Study the drawing (mm; zero at the part's minimum x, y, z) and answer. Coordinates: 2 decimals unless noted, no trailing zeros. Order: outer loops, then holes, each group sorted by start corner. A loop starts at its lowest first (then second) coordinate and runs counter-clockwise, first axis right, second up. Notation, with made-up numbers: (66.25, 87.25) - (81.25, 87.25) arc R32 cw to (81.25, 121.25) - close; hole circle Ø4 at (-36, 21.5). An arc over 180 degrees is marked (long way). Write item = value, one per line.
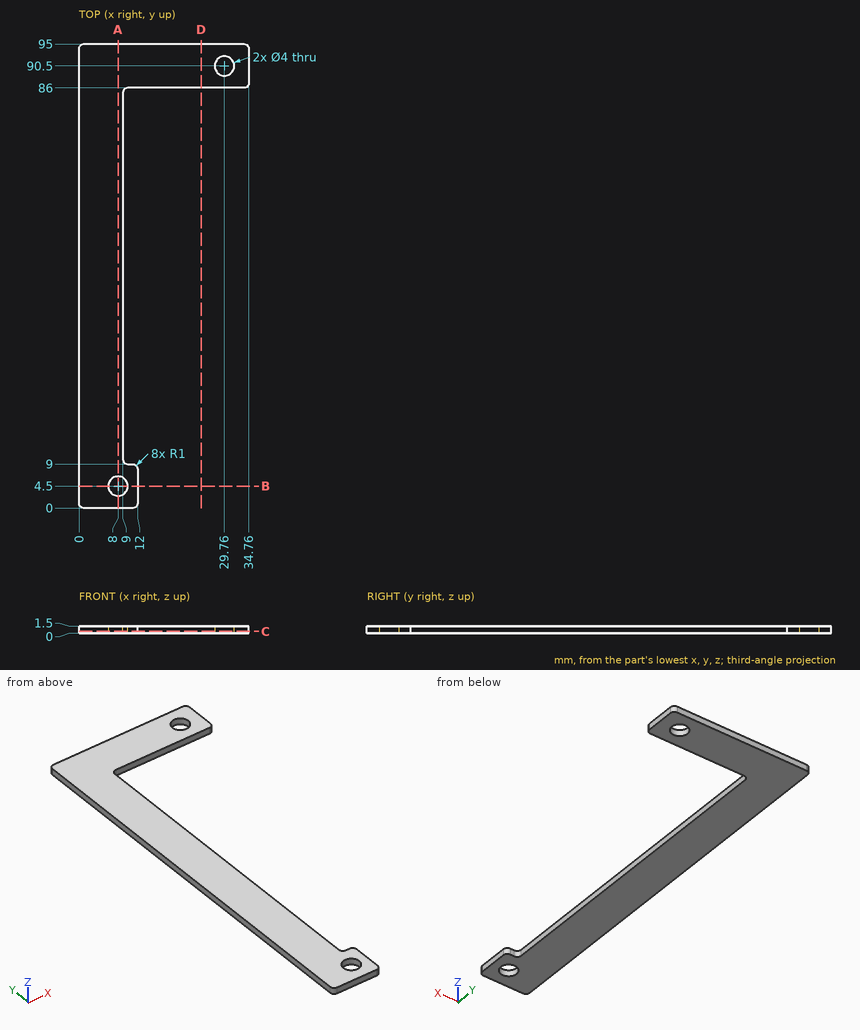
1) Straight lines are drawn through the part: line 1 along Y through (x, z) = (10.5, 0.2); line 2 along X through (y, z) = (83.5, 1.1); line 3 along Y through (x, z) = (8, 1.05). For each, find the intervals that lie inside material, in ascending order. Write a range as from..to.
Returned:
line_1 = 0..9, 86..95
line_2 = 0..9
line_3 = 0..2.5, 6.5..95
2) The part is cut by section A-A (x = 8). Determine the outline of the cut face in (y, z), and give its area (4 significant figures).
Returned:
outline = (0, 0) - (2.5, 0) - (2.5, 1.5) - (0, 1.5) - close; (6.5, 0) - (95, 0) - (95, 1.5) - (6.5, 1.5) - close
area = 136.5 mm^2
3) The part is cut by section B-B (y = 4.5). Determine the outline of the cut face in (x, z), and give its area (3 significant figures).
Returned:
outline = (0, 0) - (6, 0) - (6, 1.5) - (0, 1.5) - close; (10, 0) - (12, 0) - (12, 1.5) - (10, 1.5) - close
area = 12.0 mm^2
4) The part is cut by section D-D (x = 25). Determine the outline of the cut face in (y, z), and give its area (3 significant figures).
Returned:
outline = (86, 0) - (95, 0) - (95, 1.5) - (86, 1.5) - close
area = 13.5 mm^2
5) A flat-ended cylindrical pin translates along its axis: pin 1 Ø0.8 at (y, z) = (50, 0.5) entering from +X. Find the tip coordinate at first contact, or state that the pin passes through.
Returned:
pin_1 = 9
6) The part is cut by section C-C (z = 0.45). Determine the outline of the cut face in (x, y).
Returned:
outline = (0, 1) arc R1 ccw to (1, 0) - (11, 0) arc R1 ccw to (12, 1) - (12, 8) arc R1 ccw to (11, 9) - (10, 9) arc R1 cw to (9, 10) - (9, 85) arc R1 cw to (10, 86) - (33.76, 86) arc R1 ccw to (34.76, 87) - (34.76, 94) arc R1 ccw to (33.76, 95) - (1, 95) arc R1 ccw to (0, 94) - close; hole circle Ø4 at (8, 4.5); hole circle Ø4 at (29.76, 90.5)
